Verification items for the finished model (mm, model axes). Round coordinates to 2 decimals unless told otherwise and drop trailing zeros. Write each loop counter-clockwise with the first axis right and the second up, starting at its lowest first coordinate (ties: lowest second). Pieces come first, ordered by that corner, then holes. Notation, with made-up numbers: (23, 53.25) -> (76, 53.25) arc R25 ccw to (76, 77.25) -> close; hole circle Ø7 at (17.5, -31.75). An arc over 180 degrees is marked (long way). Use CSV: the item, a comma, the result in double quotes.
Autodesk Inventor part; units mm, degrees
ref_plane "YZ Plane" through (0, 0, 0) normal (1, 0, 0) x (0, 1, 0)
ref_plane "XZ Plane" through (0, 0, 0) normal (0, 1, 0) x (-1, 0, 0)
ref_plane "XY Plane" through (0, 0, 0) normal (0, 0, 1) x (1, 0, 0)
sketch "Sketch1" plane through (0, 0, 0) normal (0, 0, 1) x (1, 0, 0)
  circle A0 centre (0, 0) radius 5.0254
  dimension "d0" = 10.0508
extrude "Extrusion1" add sketch "Sketch1" along normal blind 202.8698
sketch "Sketch2" plane through (0, 0, 202.8698) normal (0, 0, 1) x (1, 0, 0)
  circle A0 centre (0, 0) radius 5.0254
  circle A1 centre (0, 0) radius 5.0254
  line L0 (-1.9939, 4.6129) -> (1.9939, 4.6129)
  line L1 (1.9939, 4.6129) -> (1.9939, 2.619)
  line L2 (1.9939, 2.619) -> (-1.9939, 2.619)
  line L3 (-1.9939, 2.619) -> (-1.9939, 4.6129)
  arc A2 (1.9939, 4.6129) -> (-1.9939, 4.6129) centre (0, 0) ccw
  dimension "d3" = 3.9878
  dimension "d4" = 1.9939
  dimension "d5" = 1.9939
extrude "Extrusion2" cut sketch "Sketch2" against normal blind 190.1698 contours L0 A0 | L1 L2 L3 L0
extrude "Extrusion3" add sketch "Sketch2" against normal blind 12.7 contours L0 A0 | L1 L2 L3 L0
properties part number "rod with key"
Q1. Section check C-C (z = 43). Record the cut outline in (x, y).
Filled in:
outline,"(-1.99, 2.62) -> (-1.99, 4.61) arc R5.03 ccw (long way) to (1.99, 4.61) -> (1.99, 2.62) -> close"
Q2. Mould release check, pull along Z, two halves, no side actions. Record for faces 1 (the cylindrical face through (-0.654, -4.983, 100.015)), 2 (the flat face through (0, 2.619, 103)), 3 (the flat face through (0, 0, 0)), 4 (the flat face through (0, 0, 202.87)): released by +Z, released by -Z, zero draft, split by the parting line, or undercut.
Filled in:
face 1,"zero draft"
face 2,"undercut"
face 3,"released by -Z"
face 4,"released by +Z"
Q3. Go/stop test with flat-tipped pins: P1, Ø3, axis at x = 3, z = 118.5, coming from the +Y side; P2, Ø0.6, axis at y = 3.5, z = 114.5, coming from the -X side; P3, Ø0.6, axis at y = 3.5, z = 79, coming from the +X side. Record where each tip stops, or that it passes through.
Filled in:
P1,"y = 4.61"
P2,"x = -3.87"
P3,"x = 3.87"
Q4. Material ranges on L1, parallel to X at y = -0.25, z = 52.5; L2, parallel to X at y = 4.5, z = 85.5; L3, parallel to Y at x = 0.5, z = 174.5, recorded low to high.
Filled in:
L1,"-5.02 to 5.02"
L2,"-2.24 to -1.99, 1.99 to 2.24"
L3,"-5 to 2.62"
Q5. Section check A-A (x = 0). Record the cut outline in (y, z).
Filled in:
outline,"(-5.03, 0) -> (5.03, 0) -> (5.03, 12.7) -> (2.62, 12.7) -> (2.62, 190.17) -> (5.03, 190.17) -> (5.03, 202.87) -> (-5.03, 202.87) -> close"
Q6. Section check B-B (y = -2.5). Record the cut outline in (x, z), plus the area to 3 significant figures.
Filled in:
outline,"(-4.36, 0) -> (4.36, 0) -> (4.36, 202.87) -> (-4.36, 202.87) -> close"
area,"1,770 mm²"
